The drawing under review shows one solid part. Ordinate dimensions are in mm from its lowest x, y, z. A direction names the side the tool comes from. Coordinates: 2 decimals unless noted, no trailing zeros. Order: outer loops, then holes, each group sorted by start corner. A loop starts at its lowest first (then second) coordinate and runs counter-clockwise, first axis right, second up.
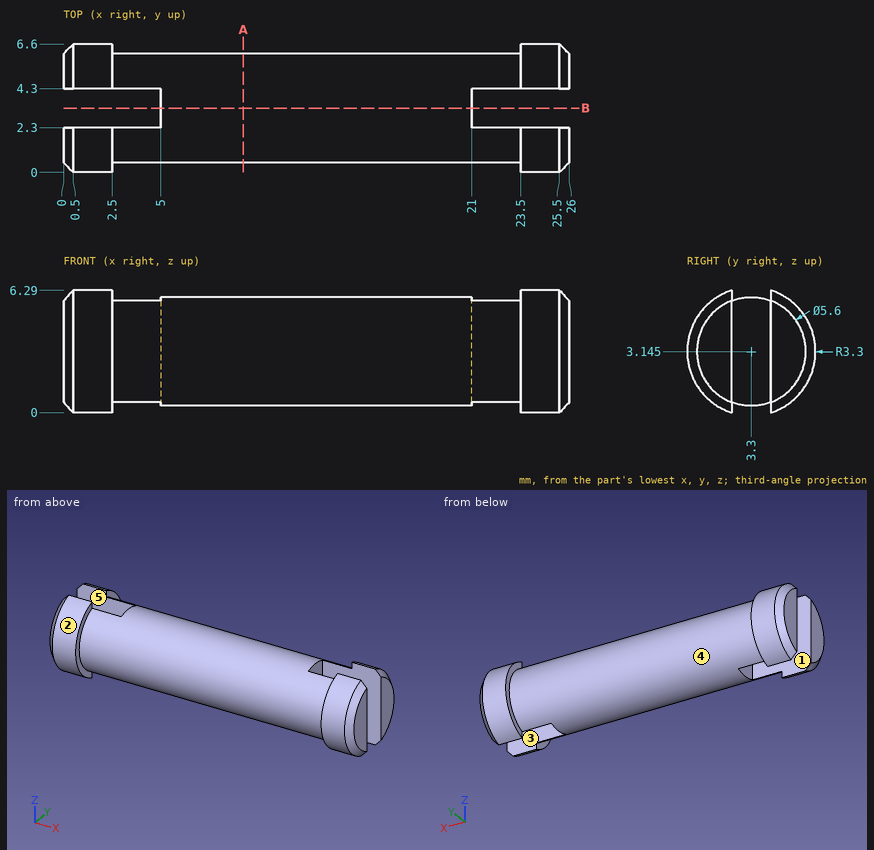
(1) Draft analysis for pull direction X (two halves, no side actions). For the marked faces 4 and 5, state which applies: released by +X, released by -X, zero draft, split by the parting line, or undercut.
A:
face 4: undercut
face 5: zero draft
(2) We need section B-B, the plane y = 3.3. Write out the cut boundary in (x, z) (1 decimal), and give its area (3 significant figures).
A:
outline: (5, 0.3) - (21, 0.3) - (21, 5.9) - (5, 5.9) - close
area: 89.6 mm2
(3) Wall thickness on probe 1 along X at (y, z) = (3.25, 0.5); probe 2 along Y at (x, z) = (16.75, 3); probe 3 along X at (y, z) = (5.5, 0.75): over which ranges is each line inside the solid? List them lowest first.
A:
probe 1: x = 5 to 21
probe 2: y = 0.5 to 6.1
probe 3: x = 0.45 to 2.5, 23.5 to 25.55
(4) Machinability: for the marked faces 1, 2 and 3, which of the approach directions +Z, -Z, +X, -X, +Y, -Y give a long, thin tool a straight path to every point of the face, cutting with its end or side? Answer none if there is none.
A:
face 1: +Z, -Z, -X
face 2: +X, -X, -Y
face 3: +Z, -Z, +X
(5) For pin 1 Ø1.5 at (x, y) = (13.5, 4.5) entering from +Z; pin 2 Ø1 at (y, z) = (3, 4) entering from +X, all flat-tipped, find the tip position at first contact; note any pin that passes through.
A:
pin 1: stops at z = 5.91
pin 2: stops at x = 21
(6) We need section A-A, the plane x = 9.25. Write out the cut boundary in (y, z) (1 decimal).
A:
outline: circle Ø5.6 at (3.3, 3.1)
